Geometry check sheet. Reference: the model listing, model coordinates, mm. A direction names the side the tool comes from. Coordinates: 2 decimals unless noted, no trailing zeros. Loops run counter-clockwise (first coordinate to the right, second up) from the corner with the lowest first, then second, coordinate; pieces in that order, holes last. Notation, with made-up numbers: (78, 87.25) -> (131, 87.25) arc R14 ccw to (131, 95.25) -> close; hole circle Ø1 at (86.25, 25). An arc over 180 degrees is marked (long way). Answer as a JSON object with one key per item and string values.
from build123d import *

# Parameters (mm, degrees)
Y_KSEKLIK_EKSTR_ZYON1_DEPTH = 60
IZIM2_R                     = 5
KES_EKSTR_ZYON1_DEPTH       = 61


with BuildPart() as part:
    # Çizim1 → Yükseklik-Ekstrüzyon1 (new body)
    with BuildSketch(Plane.XY):
        with BuildLine():
            Line((-45.299869289, 30.731722377), (-45.299869289, 28.731722377))
            ThreePointArc((-45.299869289, 28.731722377), (-46.764335383, 25.196188471), (-50.299869289, 23.731722377))
            Line((-50.299869289, 23.731722377), (-52.299869289, 23.731722377))
            ThreePointArc((-52.299869289, 23.731722377), (-54.421189632, 22.853042721), (-55.299869289, 20.731722377))
            Line((-55.299869289, 20.731722377), (-55.299869289, -13.268277623))
            ThreePointArc((-55.299869289, -13.268277623), (-54.421189632, -15.389597966), (-52.299869289, -16.268277623))
            Line((-52.299869289, -16.268277623), (-50.299869289, -16.268277623))
            ThreePointArc((-50.299869289, -16.268277623), (-46.764335383, -17.732743717), (-45.299869289, -21.268277623))
            Line((-45.299869289, -21.268277623), (-45.299869289, -23.268277623))
            ThreePointArc((-45.299869289, -23.268277623), (-44.421189632, -25.389597966), (-42.299869289, -26.268277623))
            Line((-42.299869289, -26.268277623), (-8.299869289, -26.268277623))
            ThreePointArc((-8.299869289, -26.268277623), (-6.178548945, -25.389597966), (-5.299869289, -23.268277623))
            Line((-5.299869289, -23.268277623), (-5.299869289, -21.268277623))
            ThreePointArc((-5.299869289, -21.268277623), (-3.835403195, -17.732743717), (-0.299869289, -16.268277623))
            Line((-0.299869289, -16.268277623), (1.700130711, -16.268277623))
            ThreePointArc((1.700130711, -16.268277623), (3.821451055, -15.389597966), (4.700130711, -13.268277623))
            Line((4.700130711, -13.268277623), (4.700130711, 20.731722377))
            ThreePointArc((4.700130711, 20.731722377), (3.821451055, 22.853042721), (1.700130711, 23.731722377))
            Line((1.700130711, 23.731722377), (-0.299869289, 23.731722377))
            ThreePointArc((-0.299869289, 23.731722377), (-3.835403195, 25.196188471), (-5.299869289, 28.731722377))
            Line((-5.299869289, 28.731722377), (-5.299869289, 30.731722377))
            ThreePointArc((-5.299869289, 30.731722377), (-6.178548945, 32.853042721), (-8.299869289, 33.731722377))
            Line((-8.299869289, 33.731722377), (-42.299869289, 33.731722377))
            ThreePointArc((-42.299869289, 33.731722377), (-44.421189632, 32.853042721), (-45.299869289, 30.731722377))
        make_face()
    extrude(amount=Y_KSEKLIK_EKSTR_ZYON1_DEPTH)

    # Çizim2 → Kes-Ekstrüzyon1 (cut, through all)
    with BuildSketch(Plane.XY.offset(60)):
        with Locations((-25.299869289, 3.731722377)):
            Circle(IZIM2_R)
    extrude(amount=-KES_EKSTR_ZYON1_DEPTH, mode=Mode.SUBTRACT)


solid = part.part
1. Section check A-A, the plane y = 7. Record the boundary of the cut face in (x, z), then the cut area to 3 significant figures.
Evaluation:
{"outline": "(-55.3, 0) -> (-29.08, 0) -> (-29.08, 60) -> (-55.3, 60) -> close; (-21.52, 0) -> (4.7, 0) -> (4.7, 60) -> (-21.52, 60) -> close", "area": "3,150 mm^2"}
2. Mould release check, pull along Y, two halves, no side actions. Record for faces 5 (the face through (4.7, 3, 30)), 6 (the face through (-25, 33.732, 30)), 7 (the face through (-44.44, -25.37, 29.58)), 8 (the face through (-20.53, 5.23, 30.42)): released by +Y, released by -Y, zero draft, split by the parting line, or undercut.
Evaluation:
{"face 5": "zero draft", "face 6": "released by +Y", "face 7": "released by -Y", "face 8": "undercut"}
3. Tool access check on faces 1 (the face through (-5.3, -22, 30)), 2 (the face through (-45.3, -22, 30)), 3 (the face through (-51, 23.732, 30)), 4 (the face through (1, 23.732, 30)). Record the directions out of +Z, -Z, +X, -X, +Y, -Y that give a thin tool (end or side, any length) a straight path to the whole face; none if there is none.
Evaluation:
{"face 1": "+Z, -Z, +X, -Y", "face 2": "+Z, -Z, -X, -Y", "face 3": "+Z, -Z, -X, +Y", "face 4": "+Z, -Z, +X, +Y"}
4. Depth check by flat-ended pin: P1, Ø1.6, axis at y = 29.5, z = 38, coming from the -X side; P2, Ø2, axis at y = -22.5, z = 43.5, coming from the +X side; P3, Ø0.6, axis at x = 0.5, z = 33.5, coming from the -Y side. Enter the tip coordinate at first touch or a pass-through.
Evaluation:
{"P1": "stops at x = -45.3", "P2": "stops at x = -5.3", "P3": "stops at y = -16.27"}
5. Section check B-B, the plane z = 42. Record the boundary of the cut face in (x, y), then the cut area to 3 significant figures.
Evaluation:
{"outline": "(-55.3, -13.27) arc R3 ccw to (-52.3, -16.27) -> (-50.3, -16.27) arc R5 cw to (-45.3, -21.27) -> (-45.3, -23.27) arc R3 ccw to (-42.3, -26.27) -> (-8.3, -26.27) arc R3 ccw to (-5.3, -23.27) -> (-5.3, -21.27) arc R5 cw to (-0.3, -16.27) -> (1.7, -16.27) arc R3 ccw to (4.7, -13.27) -> (4.7, 20.73) arc R3 ccw to (1.7, 23.73) -> (-0.3, 23.73) arc R5 cw to (-5.3, 28.73) -> (-5.3, 30.73) arc R3 ccw to (-8.3, 33.73) -> (-42.3, 33.73) arc R3 ccw to (-45.3, 30.73) -> (-45.3, 28.73) arc R5 cw to (-50.3, 23.73) -> (-52.3, 23.73) arc R3 ccw to (-55.3, 20.73) -> close; hole circle Ø10 at (-25.3, 3.73)", "area": "3,130 mm^2"}
6. Thickness scan on probe 1 along Y at (x, z) = (-50.5, 9.5); probe 2 along X at (y, z) = (21, 44.5); probe 3 along X at (y, z) = (31, 15). Record the ranges inside material, lowest first. Write a range as from..to.
Evaluation:
{"probe 1": "y = -16.27..23.73", "probe 2": "x = -55.29..4.69", "probe 3": "x = -45.29..-5.31"}
7. Section check C-C, the plane y = 25. Record the boundary of the cut face in (x, z), then the cut area to 3 significant figures.
Evaluation:
{"outline": "(-46.97, 0) -> (-3.63, 0) -> (-3.63, 60) -> (-46.97, 60) -> close", "area": "2,600 mm^2"}
